Read the model definition and answer for the solid it produces. Units are mm, in the model's axes. Coordinates: 2 decimals unless noted, no trailing zeros. Order: outer loops, then holes, each group sorted by start corner. A loop starts at its lowest first (then second) coordinate and runs counter-clockwise, first axis right, second up. Notation, with made-up numbers: (40.25, 8) - (81.25, 8) arc R31 ccw to (81.25, 33) - close; hole circle Ø11 at (27, -15). An arc over 180 degrees is marked (long way). Use one line per item in the form item = value.
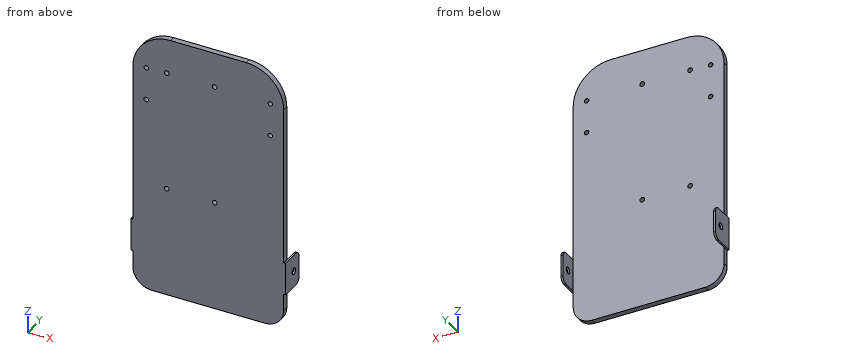
```python
from build123d import *

# Parameters (mm, degrees)
EXTRUDE_1_DEPTH        = 3
FILLET_1_R             = 20
FILLET_2_R             = 20
FILLET_3_R             = 10
SKETCH_2_R             = 1.2
CUT_EXTRUDE_1_DEPTH    = 113.548094016
SKETCH_5_W             = 1
SKETCH_5_H             = 17.3
EXTRUDE_2_DEPTH        = 10
SKETCH_7_R             = 1.7
CUT_EXTRUDE_2_DEPTH    = 133.80840887
FILLET_4_R             = 3
FILLET_4_OF_MIRROR_3_R = 3
HOLE_WIZARD_M3_1_D     = 2.5
HOLE_WIZARD_M3_1_DEPTH = 3
HOLE_WIZARD_M3_1_TIP   = 0.751075774


with BuildPart() as part:
    # 스케치1 → 보스-돌출1 (new body)
    with BuildSketch(Plane(origin=(0, 0, 0), x_dir=(1, 0, 0), z_dir=(0, 1, 0))):
        Polygon((40, -35.228470152), (-40, -35.228470152), (-40, -16.378470152), (-40, 68.621529848), (-41, 68.621529848), (-41, 85.921529848), (-40, 85.921529848), (-40, 104.771529848), (40, 104.771529848), (40, 85.921529848), (41, 85.921529848), (41, 68.621529848), (40, 68.621529848), (40, -16.378470152), align=None)
    extrude(amount=-EXTRUDE_1_DEPTH)

    # 필렛1
    fillet_1_edges = [part.edges().sort_by_distance(p)[0] for p in [
        (-40, -1.5, 35.228470152),
    ]]
    fillet(fillet_1_edges, radius=FILLET_1_R)

    # 필렛2
    fillet_2_edges = [part.edges().sort_by_distance(p)[0] for p in [
        (40, -1.5, 35.228470152),
    ]]
    fillet(fillet_2_edges, radius=FILLET_2_R)

    # 필렛3
    fillet_3_edges = [part.edges().sort_by_distance(p)[0] for p in [
        (-40, -1.5, -104.771529848),
        (40, -1.5, -104.771529848),
    ]]
    fillet(fillet_3_edges, radius=FILLET_3_R)

    # 스케치2 → 컷-돌출1 (cut, through all)
    with BuildSketch(Plane(origin=(0, 0, 0), x_dir=(1, 0, 0), z_dir=(0, 1, 0))):
        with Locations(Location((-32.87, -16.428470152, 0), (0, 0, 270))):
            Circle(SKETCH_2_R)
        with Locations(Location((-32.87, 0.971529848, 0), (0, 0, 90))):
            Circle(SKETCH_2_R)
    cut_extrude_1 = extrude(amount=-CUT_EXTRUDE_1_DEPTH, mode=Mode.SUBTRACT)

    # 대칭 복사1: 컷-돌출1 across plane
    add(cut_extrude_1.mirror(Plane(origin=(0, 0, 0), x_dir=(0, 0, 1), z_dir=(1, 0, 0))), mode=Mode.SUBTRACT)

    # 스케치5 → 보스-돌출2 (add)
    with BuildSketch(Plane(origin=(0, 0, 0), x_dir=(1, 0, 0), z_dir=(0, 1, 0))):
        with Locations((-40.5, 77.271529848)):
            Rectangle(SKETCH_5_W, SKETCH_5_H)
    extrude_2 = extrude(amount=EXTRUDE_2_DEPTH)

    # 스케치7 → 컷-돌출2 (cut, through all)
    with BuildSketch(Plane(origin=(-40, 0, 0), x_dir=(0, 0, -1), z_dir=(1, 0, 0))):
        with Locations((77.271529848, 5)):
            Circle(SKETCH_7_R)
    cut_extrude_2 = extrude(amount=-CUT_EXTRUDE_2_DEPTH, mode=Mode.SUBTRACT)

    # 필렛4
    fillet_4_edges = [part.edges().sort_by_distance(p)[0] for p in [
        (-40.5, 10, -68.621529848),
        (-40.5, 10, -85.921529848),
    ]]
    fillet(fillet_4_edges, radius=FILLET_4_R)

    # 대칭 복사3: 보스-돌출2, 컷-돌출2 across plane
    add(extrude_2.mirror(Plane(origin=(0, 0, 0), x_dir=(0, 0, 1), z_dir=(1, 0, 0))))
    add(cut_extrude_2.mirror(Plane(origin=(0, 0, 0), x_dir=(0, 0, 1), z_dir=(1, 0, 0))), mode=Mode.SUBTRACT)

    # 필렛4 of 대칭 복사3
    fillet_4_of_mirror_3_edges = [part.edges().sort_by_distance(p)[0] for p in [
        (40.5, 10, -68.621529848),
        (40.5, 10, -85.921529848),
    ]]
    fillet(fillet_4_of_mirror_3_edges, radius=FILLET_4_OF_MIRROR_3_R)

    # M3 탭을 위한 탭 드릴1
    with Locations(Plane(origin=(0, 0, 0), x_dir=(1, 0, 0), z_dir=(0, 1, 0))):
        with Locations((-22, -16.800227959), (3.4, -16.800227959), (3.4, 46.699772041), (-22, 46.699772041)):
            Hole(HOLE_WIZARD_M3_1_D / 2, depth=HOLE_WIZARD_M3_1_DEPTH)
            with Locations((0, 0, -(HOLE_WIZARD_M3_1_DEPTH + HOLE_WIZARD_M3_1_TIP / 2))):  # 118° drill point
                Cone(0, HOLE_WIZARD_M3_1_D / 2, HOLE_WIZARD_M3_1_TIP, mode=Mode.SUBTRACT)


solid = part.part
```
(1) Section C-C, the plane x = -6 is taken. Write down the section's boundary in (y, z), then the cut area to 3 significant figures.
Answer list:
outline = (-3, -104.77) - (0, -104.77) - (0, 35.23) - (-3, 35.23) - close
area = 420 mm2
(2) Given pin 1 Ø3.5 at (y, z) = (-2, -27.5) entering from +X; pin 2 Ø4 at (x, z) = (-32.87, -0.97) entering from -Y; pin 3 Ø3 at (x, z) = (32.87, 16.43) entering from +Y; pin 4 Ø0.8 at (x, y) = (-40.5, 0) entering from +Z, each flat-ended and moving along its own axis, determine where each tip first touches the part or whether it passes through.
Answer list:
pin_1 = 40
pin_2 = -3
pin_3 = 0
pin_4 = -68.62
(3) Section A-A, the plane y = 1.5 is taken. Write down the section's boundary in (x, z).
Answer list:
outline = (-41, -85.92) - (-40, -85.92) - (-40, -68.62) - (-41, -68.62) - close; (40, -85.92) - (41, -85.92) - (41, -68.62) - (40, -68.62) - close
(4) Straight lines are drawn through the part: L1, parallel to Z at x = 3.4, y = -1.7; L2, parallel to X at y = 2, z = -85; L3, parallel to Z at x = 32.87, y = -1.1. For each, find the intervals that lie inside material, in ascending order.
Answer list:
L1 = -104.77 to -47.95, -45.45 to 15.55, 18.05 to 35.23
L2 = -41 to -40, 40 to 41
L3 = -104.35 to -2.17, 0.23 to 15.23, 17.63 to 30.54
(5) Section B-B, the plane z = -42.5 is taken. Write down the section's boundary in (x, y).
Answer list:
outline = (-40, -3) - (40, -3) - (40, 0) - (-40, 0) - close
